Could you check a few things on this model? Use its own coordinates, in mm. A direction names the side the tool comes from. Give positions to 0.01 mm unless a question says otherwise; leave off trailing zeros. Loops run counter-clockwise (first coordinate to the right, second up) from the corner with the lowest first, then second, coordinate; pieces in that order, holes last. Notation, with made-up numbers: (50.25, -35.75) -> (60.25, -35.75) arc R17 ccw to (60.25, -29.75) -> close; hole circle Ø3 at (40.5, 7.25). An arc over 180 degrees is marked (long way). Put each result on its own line as item: value.
```python
from build123d import *

# Parameters (mm, degrees)
F1_DEPTH      = 12.5
F2_DEPTH      = 300
F2_DEPTH_BACK = 12.5
F0_R          = 6
F3_DEPTH      = 50
F4_R          = 0.5


# Not quite as in the source:
# - a feature names something its author has since deleted; it is built from what else it names


with BuildPart() as f1:
    # F0 (on Top) → F1 (new body, symmetric)
    with BuildSketch(Plane.XY):
        with BuildLine():
            Line((-15, 50), (-65, 50))
            ThreePointArc((-65, 50), (-72.0710678119, 47.0710678119), (-75, 40))
            Line((-75, 40), (-75, -40))
            ThreePointArc((-75, -40), (-72.0710678119, -47.0710678119), (-65, -50))
            Line((-65, -50), (65, -50))
            ThreePointArc((65, -50), (72.0710678119, -47.0710678119), (75, -40))
            Line((75, -40), (75, 40))
            ThreePointArc((75, 40), (72.0710678119, 47.0710678119), (65, 50))
            Line((65, 50), (15, 50))
            Line((15, 50), (2.5, 50))
            Line((2.5, 50), (2.5, 40.0037090484))
            Line((2.5, 40.0037090484), (65, 40.0037090484))
            Line((65, 40.0037090484), (65, -40.0037090484))
            Line((65, -40.0037090484), (-65, -40.0037090484))
            Line((-65, -40.0037090484), (-65, 40.0037090484))
            Line((-65, 40.0037090484), (-2.5, 40.0037090484))
            Line((-2.5, 40.0037090484), (-2.5, 50))
            Line((-2.5, 50), (-15, 50))
        make_face()
        Polygon((2.5, 50), (-2.5, 50), (-2.5, 40.0037090484), (0, 40.0037090484), (2.5, 40.0037090484), align=None)
    extrude(amount=F1_DEPTH, both=True)

    # F0 (on Top) → F2 (join, two sides)
    with BuildSketch(Plane.XY) as f2_sk:
        Polygon((-15, 80), (-15, 50), (-2.5, 50), (-2.5, 53.9933157269), (-9, 53.9933157269), (-9, 76.9933157269), (0, 76.9933157269), (0, 79.2549662558), (0, 80), align=None)
        Polygon((2.5, 53.9933157269), (2.5, 50), (15, 50), (15, 80), (0, 80), (0, 79.2549662558), (0, 76.9933157269), (9, 76.9933157269), (9, 53.9933157269), align=None)
    extrude(amount=F2_DEPTH)
    extrude(f2_sk.sketch, amount=-F2_DEPTH_BACK)

    # F0 (on Top) → F3 (cut)
    with BuildSketch(Plane.XY):
        with Locations((0, 69.7)):
            Circle(F0_R)
    extrude(amount=F3_DEPTH, mode=Mode.SUBTRACT)

    # F4
    f4_edges = [f1.edges().sort_by_distance(p)[0] for p in [
        (-9, 76.993316, 143.75),
        (9, 76.993316, 143.75),
        (-9, 53.993316, 143.75),
        (9, 53.993316, 143.75),
    ]]
    fillet(f4_edges, radius=F4_R)


solid = f1.part
```
1. I need wall thicknesses on line 1 (X direction, y = 53.5, z = 136.5); line 2 (X direction, y = 71, z = 127); line 3 (Z direction, x = 59.5, y = -44). Which ranges of each line are inside material? Lowest first, please.
Recorded:
line 1: x = -15 to -2.5, 2.5 to 15
line 2: x = -15 to -9, 9 to 15
line 3: z = -12.5 to 12.5
2. If we section it at B-B (x = 58): List the corners of the cut face in (y, z) for me.
Recorded:
outline: (-50, -12.5) -> (-40, -12.5) -> (-40, 12.5) -> (-50, 12.5) -> close; (40, -12.5) -> (50, -12.5) -> (50, 12.5) -> (40, 12.5) -> close
3. If we section it at C-C (z = 257): List the corners of the cut face in (x, y) for me, then the cut area to 3 significant figures.
Recorded:
outline: (-15, 50) -> (-2.5, 50) -> (-2.5, 53.99) -> (-8.5, 53.99) arc R0.5 cw to (-9, 54.49) -> (-9, 76.49) arc R0.5 cw to (-8.5, 76.99) -> (8.5, 76.99) arc R0.5 cw to (9, 76.49) -> (9, 54.49) arc R0.5 cw to (8.5, 53.99) -> (2.5, 53.99) -> (2.5, 50) -> (15, 50) -> (15, 80) -> (-15, 80) -> close
area: 466 mm^2
4. If we section it at D-D (z = 9): List the corners of the cut face in (x, y) for me, then the cut area to 3 significant figures.
Recorded:
outline: (-75, -40) arc R10 ccw to (-65, -50) -> (65, -50) arc R10 ccw to (75, -40) -> (75, 40) arc R10 ccw to (65, 50) -> (15, 50) -> (15, 80) -> (-15, 80) -> (-15, 50) -> (-65, 50) arc R10 ccw to (-75, 40) -> close; hole (-65, -40) -> (65, -40) -> (65, 40) -> (-65, 40) -> close; hole (-9, 54.49) arc R0.5 ccw to (-8.5, 53.99) -> (-2.5, 53.99) -> (-2.5, 50) -> (2.5, 50) -> (2.5, 53.99) -> (8.5, 53.99) arc R0.5 ccw to (9, 54.49) -> (9, 76.49) arc R0.5 ccw to (8.5, 76.99) -> (-8.5, 76.99) arc R0.5 ccw to (-9, 76.49) -> close
area: 4,980 mm^2
5. For faces 4 (the face through (6, 53.993, 146)), 5 (the face through (-9, 50, 154)), 6 (the face through (0, 80, 146)), which set-ups out of +Z, -Z, +X, -X, +Y, -Y let a thin tool reach every point of the face, with its end or its side?
Recorded:
face 4: +Z, -Z
face 5: +Z, +X, -X, -Y
face 6: +Z, -Z, +X, -X, +Y
6. Thinking about a two-plate mould opening in Y: for faces 1 (the face through (0, 76.993, 146)), 2 (the face through (-15, 65, 146)), 3 (the face through (40, 50, 0)), which applies, pulls with the +Y half, pulls with the -Y half, needs draft (parallel to the pull), parting line crosses it, or undercut?
Recorded:
face 1: undercut
face 2: needs draft
face 3: pulls with the +Y half
7. I'm going to push flat-ended pins straight in: pin 1 (12.5 mm diameter, centred on x = 36, z = -4.5, fed in from +Y); pin 2 (6.5 mm diameter, centred on y = 69, z = 192, fed in from +X); pin 3 (11 mm diameter, centred on y = 64.5, z = 151.5, fed in from -X). Where does each tip first touch, or does it pass through?
Recorded:
pin 1: stops at y = 50
pin 2: stops at x = 15
pin 3: stops at x = -15
8. If we section it at A-A (y = 70): List the corners of the cut face in (x, z) for me, then the cut area to 3 significant figures.
Recorded:
outline: (-15, -12.5) -> (-9, -12.5) -> (-9, 300) -> (-15, 300) -> close; (9, -12.5) -> (15, -12.5) -> (15, 300) -> (9, 300) -> close
area: 3,750 mm^2
